Autodesk Inventor part; units mm, degrees
ref_plane "YZ Plane" through (0, 0, 0) normal (1, 0, 0) x (0, 1, 0)
ref_plane "XZ Plane" through (0, 0, 0) normal (0, 1, 0) x (-1, 0, 0)
ref_plane "XY Plane" through (0, 0, 0) normal (0, 0, 1) x (1, 0, 0)
sketch "スケッチ1" plane through (0, 0, 0) normal (0, 0, 1) x (1, 0, 0)
  circle A0 centre (0, 0) radius 65
  circle A1 centre (0, 0) radius 55
  circle A2 centre (0, 0) radius 25
  line L0 (0, 0) -> (0, 65)
  circle A3 centre (0, 0) radius 6.05
  line L1 (5, 0) -> (5, 64.8074)
  line L2 (5, 0) -> (69.8074, 0) construction
  line L3 (-5, 0) -> (-5, 64.8074)
  line L4 (-2.5, -4.3301) -> (-58.6249, 28.0736)
  line L5 (2.5, 4.3301) -> (-53.6249, 36.7338)
  line L6 (2.5, -4.3301) -> (-53.6249, -36.7338)
  line L7 (-2.5, 4.3301) -> (-58.6249, -28.0736)
  line L8 (5, 0) -> (5, -64.8074)
  line L9 (-5, 0) -> (-5, -64.8074)
  line L10 (2.5, 4.3301) -> (58.6249, -28.0736)
  line L11 (-2.5, -4.3301) -> (53.6249, -36.7338)
  line L12 (-2.5, 4.3301) -> (53.6249, 36.7338)
  line L13 (2.5, -4.3301) -> (58.6249, 28.0736)
  circle A4 centre (0, 0) radius 72.5
  line L14 (0, 0) -> (36.25, 62.7868)
  line L15 (0, 0) -> (72.5, 0) construction
  line L16 (0, 0) -> (30.6398, 65.7073)
  line L17 (0, 0) -> (72.5, 0) construction
  line L18 (0, 0) -> (41.5843, 59.3885)
  line L19 (0, 0) -> (72.5, 0) construction
  line L20 (0, 65) -> (0, 72.5)
  circle A5 centre (0, 0) radius 69.5
  circle A6 centre (0, 0) radius 64.5
  circle A7 centre (26.0299, 61.7369) radius 2.5
  line L21 (0, 0) -> (-30.6398, 65.7073)
  circle A8 centre (-26.0299, 61.7369) radius 2.5
  circle A9 centre (-40.4507, 53.411) radius 2.5
  circle A10 centre (-66.4807, 8.3259) radius 2.5
  circle A11 centre (-66.4807, -8.3259) radius 2.5
  circle A12 centre (-40.4507, -53.411) radius 2.5
  circle A13 centre (-26.0299, -61.7369) radius 2.5
  circle A14 centre (26.0299, -61.7369) radius 2.5
  circle A15 centre (40.4507, -53.411) radius 2.5
  circle A16 centre (66.4807, -8.3259) radius 2.5
  circle A17 centre (66.4807, 8.3259) radius 2.5
  circle A18 centre (40.4507, 53.411) radius 2.5
  point P0 (5, 54.7723)
  point P1 (44.9342, 31.7163)
  point P2 (18.7132, 16.5776)
  point P3 (5, 24.4949)
  point P4 (-5, 54.7723)
  point P5 (-5, 24.4949)
  point P6 (-18.7132, 16.5776)
  point P7 (-44.9342, 31.7163)
  point P8 (49.9342, -23.056)
  point P9 (23.7132, -7.9173)
  point P10 (23.7132, 7.9173)
  point P11 (49.9342, 23.056)
  point P12 (5, -54.7723)
  point P13 (5, -24.4949)
  point P14 (18.7132, -16.5776)
  point P15 (44.9342, -31.7163)
  point P16 (-44.9342, -31.7163)
  point P17 (-18.7132, -16.5776)
  point P18 (-5, -24.4949)
  point P19 (-5, -54.7723)
  point P20 (-49.9342, 23.056)
  point P21 (-23.7132, 7.9173)
  point P22 (-23.7132, -7.9173)
  point P23 (-49.9342, -23.056)
  point P24 (27.4702, 58.91)
  point P25 (28.2957, 60.6803)
  point P26 (25.0587, 59.4333)
  point P27 (-25.0587, 59.4333)
  point P28 (-28.2957, 60.6803)
  point P29 (-27.4702, 58.91)
  point P30 (-26.6077, 59.3046)
  point P31 (-27.0012, 64.0405)
  point P32 (27.0012, 64.0405)
  point P33 (26.6077, 59.3046)
  point P34 (37.2825, 53.2449)
  point P35 (-64.0001, 8.0152)
  point P36 (-68.9613, 8.6365)
  point P37 (-41.9601, 55.404)
  point P38 (-38.9414, 51.4181)
  point P39 (25.0587, -59.4333)
  point P40 (27.0012, -64.0405)
  point P41 (-27.0012, -64.0405)
  point P42 (-25.0587, -59.4333)
  point P43 (38.9414, 51.4181)
  point P44 (41.9601, 55.404)
  point P45 (68.9613, 8.6365)
  point P46 (64.0001, 8.0152)
  point P47 (64.0001, -8.0152)
  point P48 (68.9613, -8.6365)
  point P49 (41.9601, -55.404)
  point P50 (38.9414, -51.4181)
  point P51 (-38.9414, -51.4181)
  point P52 (-41.9601, -55.404)
  point P53 (-68.9613, -8.6365)
  point P54 (-64.0001, -8.0152)
  dimension "d0" = 130
  dimension "d1" = 110
  dimension "d2" = 50
  dimension "d3" = 12.1
  dimension "d4" = 90
  dimension "d7" = 360
  dimension "d36" = 145
  dimension "d37" = 72.5
  dimension "d38" = 60
  dimension "d39" = 65
  dimension "d40" = 55
  dimension "d41" = 139
  dimension "d42" = 129
  dimension "d43" = 5
  dimension "d50" = 360
extrude "押し出し1" add sketch "スケッチ1" along normal blind 2 contours A6 L10 A1 L13 | L13 A1 L12 A6 | L12 A1 L18 A6 | A17 A5 A16 A0 | A0 A16 A6 A17 | A5 L18 A4 L21 | L13 A2 L12 A1 | A18 A6 L18 A0 | A0 L18 A18 | A18 L18 A5 | L13 L10 A3 L1 L18 L12 A2 | A2 L10 L13 | L18 A6 L14 A0 | A0 L14 A5 L18 | L18 A1 L14 A6 | L12 L18 A2 | A5 L14 A4 L18 | L10 A6 L11 A1 | A1 L11 A2 L10 | L13 A3 L10 | L10 A2 L11 L8 A3 L13 | L14 A6 L16 A0 | A0 L16 A5 L14 | L14 A1 L16 A6 | L18 L12 L14 A2 | L18 L1 L12 | A5 A14 A0 A15 | A5 L16 A4 L14 | L11 A6 L8 A1 | L16 A6 A7 A0 | A0 A7 L16 | L16 A1 L1 A6 | L14 L1 L16 A2 | L12 L16 L1 | L14 A3 L16 L12 | L1 L18 A3 L14 | L1 A3 L18 | A0 A14 A6 A15 | A5 L20 A4 L16 | L16 A7 A5 | L8 A6 L9 A1 | A1 L9 A2 L8 | A2 L8 L11 | L8 L11 A3 | L1 A2 L0 A1 | A1 L0 A6 L1 | L16 L1 A2 | L16 L12 A3 L0 A2 L1 | L16 A3 L12 | A5 A12 A0 A13 | A4 L20 A5 L21 | L9 A6 L6 A1 | A2 L9 L6 A3 L11 L8 | L0 A2 L3 A1 | A1 L3 A6 L0 | A0 A12 A6 A13 | L21 A0 A9 A5 | A5 A8 L21 | L6 A6 L7 A1 | A1 L7 A2 L6 | A2 L6 L9 | L6 L9 A3 | A1 L21 A6 L3 | L0 A3 L5 L21 L3 A2 | A5 A10 A0 A11 | A8 A0 L21 | L7 A6 L4 A1 | A2 L7 L4 A3 L9 L6 | A1 L5 A6 L21 | L3 L21 A2 | A3 L21 L5 | A0 A10 A6 A11 | L21 A6 A9 A0 | A0 A8 A6 L21 | L4 A6 L5 A1 | A1 L5 A2 L4 | A2 L4 L7 | A3 L3 L5 L21 | L4 L7 A3 | L21 L3 L5 A2 | L21 L5 L3 | A2 L5 L3 A3 L7 L4
sketch "スケッチ2" plane through (0, 0, 2) normal (0, 0, 1) x (1, 0, 0)
  point P0 (0, 0)
  point P1 (0, 18)
  point P2 (-18, 0)
  point P3 (0, -18)
  point P4 (18, 0)
  point P5 (0, 55)
  point P6 (-47.6314, 27.5)
  point P7 (-47.6314, -27.5)
  point P8 (0, -55)
  point P9 (47.6314, -27.5)
  point P10 (47.6314, 27.5)
  dimension "d11" = 18
  dimension "d14" = 360
  dimension "d16" = 55
  dimension "d19" = 360
hole "穴1" at (0, 18, 2) at (-18, 0, 2) at (0, -18, 2) at (18, 0, 2) direction (0, 0, -1) diameter 4 end through all
hole "穴2" at (0, 55, 2) at (-47.6314, 27.5, 2) at (-47.6314, -27.5, 2) at (0, -55, 2) at (47.6314, -27.5, 2) at (47.6314, 27.5, 2) direction (0, 0, -1) diameter 3.2 end through all
fillet "フィレット1" radius 6 24 edges at (-49.9342, 23.056, 1) (-49.9342, -23.056, 1) (-23.7132, -7.9173, 1) (-23.7132, 7.9173, 1) (-44.9342, 31.7163, 1) (-18.7132, 16.5776, 1) (-5, 24.4949, 1) (-5, 54.7723, 1) (5, 54.7723, 1) (5, 24.4949, 1) (18.7132, 16.5776, 1) (44.9342, 31.7163, 1) (49.9342, 23.056, 1) (23.7132, 7.9173, 1) (23.7132, -7.9173, 1) (49.9342, -23.056, 1) (44.9342, -31.7163, 1) (18.7132, -16.5776, 1) (5, -24.4949, 1) (5, -54.7723, 1) (-5, -54.7723, 1) (-5, -24.4949, 1) (-18.7132, -16.5776, 1) (-44.9342, -31.7163, 1)
properties part number "TH22_tire_3rd_POM" material "アルミニウム 6061-AHC"
Design review of the part built by this model. Coordinates are the model's own, in mm. Coordinates: 2 decimals unless noted, no trailing zeros. Loops run counter-clockwise (first coordinate to the right, second up) from the corner with the lowest first, then second, coordinate; pieces in that order, holes last.
Item 1: Add section C-C (x = -59). Write out the cut boundary in (y, z).
Completed:
outline: (-42.13, 0) - (-36.73, 0) - (-36.73, 2) - (-42.13, 2) - close; (-26.06, 0) - (26.06, 0) - (26.06, 2) - (-26.06, 2) - close; (36.73, 0) - (42.13, 0) - (42.13, 2) - (36.73, 2) - close
Item 2: Draft analysis for pull direction Y (two halves, no side actions). For faces 1 (the cylindrical face through (59.99, 35.09, 0.99)), 2 (the flat face through (30.612, -23.447, 0.986)), 3 (the cylindrical face through (69.15, -21.78, 0.99)), state which applies: pulls with the +Y half, pulls with the -Y half, needs draft (parallel to the pull), parting line crosses it, or undercut.
Completed:
face 1: undercut
face 2: undercut
face 3: parting line crosses it
Item 3: Add section B-B (x = 18). Write out the cut boundary in (y, z).
Completed:
outline: (-70.23, 0) - (-67.13, 0) - (-67.13, 2) - (-70.23, 2) - close; (-61.94, 0) - (-51.97, 0) - (-51.97, 2) - (-61.94, 2) - close; (-18.23, 0) - (-2, 0) - (-2, 2) - (-18.23, 2) - close; (2, 0) - (18.23, 0) - (18.23, 2) - (2, 2) - close; (51.97, 0) - (61.94, 0) - (61.94, 2) - (51.97, 2) - close; (67.13, 0) - (70.23, 0) - (70.23, 2) - (67.13, 2) - close
Item 4: Clearance check with flat-ended pins moving along their axes: pin 1 (1 mm diameter, centred on y = -40, z = 1, fed in from -X); pin 2 (1 mm diameter, centred on y = 37, z = 1, fed in from +X); pin 3 (0.6 mm diameter, centred on y = 36, z = 0.5, fed in from -X). State where each tip first meets the part, or that it passes through.
Completed:
pin 1: stops at x = -60.79
pin 2: stops at x = 62.64
pin 3: stops at x = -63.1
Item 5: Add section A-A (y = 0). Write out the cut boundary in (x, z).
Completed:
outline: (-72.5, 0) - (-55, 0) - (-55, 2) - (-72.5, 2) - close; (-25, 0) - (-20, 0) - (-20, 2) - (-25, 2) - close; (-16, 0) - (-6.05, 0) - (-6.05, 2) - (-16, 2) - close; (6.05, 0) - (16, 0) - (16, 2) - (6.05, 2) - close; (20, 0) - (25, 0) - (25, 2) - (20, 2) - close; (55, 0) - (72.5, 0) - (72.5, 2) - (55, 2) - close
Item 6: Wall thickness on L1, parallel to Y at x = 37, z = 0.9; L2, parallel to X at y = 55, z = 1.25; L3, parallel to Y at x = -24, z = 1.65: over which ranges is each line inside the solid? List them lowest first.
Completed:
L1: y = -62.35 to -40.69, -27.14 to -15.59, 15.59 to 27.14, 40.69 to 62.35
L2: x = -47.24 to -42.49, -38.52 to -1.6, 1.6 to 38.52, 42.49 to 47.24
L3: y = -68.41 to -65.22, -59.87 to -49.49, -19.63 to 19.63, 49.49 to 59.87, 65.22 to 68.41
Item 7: Add section D-D (z = 0.7). Give the number of separate pieces and of enclosed holes in the cut face, and give its area (3 significant figures).
Completed:
separate pieces: 1
enclosed holes: 23
area: 9,030 mm2
